Work out the finished part from the listing and answer in its coordinate system (mm). Coordinates: 2 decimals unless noted, no trailing zeros. Answer as CSV lines item,"result". Start each with the question number.
(1) A flat-ended cylindrical pin translates along its axis: P1, Ø1.5, axis at x = 52.5, y = -10, coming from the -Z side. Find the tip coordinate at first contact, or state that the pin passes through.
(2) The mould has two halves that part along Y. Classify faces 1 (the cylindrical face through (79.34, 71.33, 5.07)), 2 (the flat face through (2, 4, 0)): released by +Y, released by -Y, zero draft, split by the parting line, or undercut.
(3) Find the intervals of material crossed by L1, parallel to Y at x = -70.5, z = 3.5; L2, parallel to Y at x = -41, z = 9; L3, parallel to X at y = 13, z = 7, in increasing order. Write a range as [from, to].
(4) A cutting plane is placed at A-A on z = 1.75. Count the separate pieces of the cut face and the enclosed holes in it, then the cut area to 3 significant figures.
from build123d import *

# Parameters (mm, degrees)
F0_W     = 240
F0_H     = 150
F1_DEPTH = 10
F2_D     = 6.6
F3_D     = 6.6
F4_D     = 5.5
F5_D     = 5.5


with BuildPart() as f1:
    # F0 (on Top) → F1 (new body)
    with BuildSketch(Plane.XY):
        with Locations((3.8884611577, 2.5630567968)):
            Rectangle(F0_W, F0_H)
    extrude(amount=F1_DEPTH)

    # F2 (through all)
    with Locations(Plane(origin=(0, 0, 0), x_dir=(1, 0, 0), z_dir=(0, 0, -1))):
        with Locations((-7.6115388423, 29.9369432032), (-42.6115388423, -35.0630567968), (-42.6115388423, 29.9369432032), (-42.6115388423, 64.9369432032), (-7.6115388423, -35.0630567968), (-42.6115388423, -70.0630567968), (82.3884611577, -35.0630567968), (-7.6115388423, -70.0630567968), (82.3884611577, 29.9369432032), (82.3884611577, 64.9369432032), (117.3884611577, 29.9369432032), (117.3884611577, -35.0630567968), (82.3884611577, -70.0630567968), (117.3884611577, -70.0630567968), (117.3884611577, 64.9369432032), (-7.6115388423, 64.9369432032)):
            Hole(F2_D / 2)

    # F3 (through all)
    with Locations(Plane(origin=(0, 0, 0), x_dir=(1, 0, 0), z_dir=(0, 0, -1))):
        with Locations((-70.1115388423, 32.4369432032), (-70.1115388423, 67.4369432032), (-70.1115388423, -72.5630567968), (-105.1115388423, -37.5630567968), (-105.1115388423, -72.5630567968), (-105.1115388423, 67.4369432032), (-105.1115388423, 32.4369432032), (-70.1115388423, -37.5630567968), (19.8884611577, -72.5630567968), (54.8884611577, -72.5630567968), (54.8884611577, -37.5630567968), (19.8884611577, -37.5630567968), (54.8884611577, 32.4369432032), (19.8884611577, 67.4369432032), (54.8884611577, 67.4369432032), (19.8884611577, 32.4369432032)):
            Hole(F3_D / 2)

    # F4 (through all)
    with Locations(Plane(origin=(0, 0, 0), x_dir=(1, 0, 0), z_dir=(0, 0, -1))):
        with Locations((17.3884611577, -14.5630567968), (17.3884611577, 9.4369432032), (57.3884611577, 9.4369432032), (57.3884611577, -14.5630567968)):
            Hole(F4_D / 2)

    # F5 (through all)
    with Locations(Plane(origin=(0, 0, 0), x_dir=(1, 0, 0), z_dir=(0, 0, -1))):
        with Locations((-108.1115388423, -22.5630567968), (-84.1115388423, -22.5630567968), (-108.1115388423, 17.4369432032), (-84.1115388423, 17.4369432032)):
            Hole(F5_D / 2)


solid = f1.part
Here are the results:
1,P1,"stops at z = 0"
2,face 1,"undercut"
2,face 2,"zero draft"
3,L1,"y = [-72.44, -70.71], [-64.16, -35.71], [-29.16, 34.29], [40.84, 69.29], [75.84, 77.56]"
3,L2,"y = [-72.44, -67.82], [-62.06, -32.82], [-27.06, 32.18], [37.94, 67.18], [72.94, 77.56]"
3,L3,"x = [-116.11, 15.13], [19.65, 55.13], [59.65, 123.89]"
4,separate pieces,"1"
4,enclosed holes,"40"
4,area,"34,700 mm^2"
